```python
from build123d import *

# Parameters (mm, degrees)
SKETCH_1_W          = 80
SKETCH_1_H          = 36
EXTRUDE_1_DEPTH     = 2
CUT_EXTRUDE_1_DEPTH = 2
FILLET_2_R          = 2
SKETCH_3_R          = 1.5
CUT_EXTRUDE_2_DEPTH = 44.9089968


with BuildPart() as part:
    # 草图1 → 凸台-拉伸1 (new body)
    with BuildSketch(Plane.XY):
        Rectangle(SKETCH_1_W, SKETCH_1_H)
    extrude(amount=EXTRUDE_1_DEPTH)

    # 草图2 → 切除-拉伸1 (cut)
    with BuildSketch(Plane.XY.offset(2)):
        Polygon((-30, -8), (-30, -13), (30, -13), (30, -8), (30, 8), (30, 13), (-30, 13), (-30, 8), align=None)
    extrude(amount=-CUT_EXTRUDE_1_DEPTH, mode=Mode.SUBTRACT)

    # 圆角2
    fillet_2_edges = [part.edges().sort_by_distance(p)[0] for p in [
        (30, -13, 1),
        (-30, -13, 1),
        (-30, 13, 1),
        (30, 13, 1),
    ]]
    fillet(fillet_2_edges, radius=FILLET_2_R)

    # 草图3 → 切除-拉伸2 (cut, through all)
    with BuildSketch(Plane.XY.offset(2)):
        with Locations((23, -15)):
            Circle(SKETCH_3_R)
        with Locations((13, -15)):
            Circle(SKETCH_3_R)
        with Locations((-13, -15)):
            Circle(SKETCH_3_R)
        with Locations((-23, -15)):
            Circle(SKETCH_3_R)
        with Locations((23, 15)):
            Circle(SKETCH_3_R)
        with Locations((13, 15)):
            Circle(SKETCH_3_R)
        with Locations((-13, 15)):
            Circle(SKETCH_3_R)
        with Locations((-23, 15)):
            Circle(SKETCH_3_R)
    extrude(amount=-CUT_EXTRUDE_2_DEPTH, mode=Mode.SUBTRACT)


solid = part.part
```
Design review of the part built by this model. Coordinates are the model's own, in mm. A direction names the side the tool comes from. Coordinates: 2 decimals unless noted, no trailing zeros. Loops run counter-clockwise (first coordinate to the right, second up) from the corner with the lowest first, then second, coordinate; pieces in that order, holes last.
Q1. Tool access review of faces 4 (the face through (-29.4, -12.43, 0.99)), 5 (the face through (-1, -16, 0)): name each direction out of +Z, -Z, +X, -X, +Y, -Y from which nothing blocks a thin tool from reaching the whole face with its end or side.
Reported:
face 4: +Z, -Z
face 5: -Z, +X, -X, +Y, -Y
Q2. To check wall thickness, follow line 1 (Y direction, x = 13, z = 0.55); line 2 (Y direction, x = 27, z = 1.35); line 3 (X direction, y = -7, z = 1.3). State the ranges of each line that lie inside material, in increasing order.
Reported:
line 1: y = -18 to -16.5, -13.5 to -13, 13 to 13.5, 16.5 to 18
line 2: y = -18 to -13, 13 to 18
line 3: x = -40 to -30, 30 to 40
Q3. We need section D-D on y = -15. State the section outline as (x, z) points.
Reported:
outline: (-40, 0) - (-24.5, 0) - (-24.5, 2) - (-40, 2) - close; (-21.5, 0) - (-14.5, 0) - (-14.5, 2) - (-21.5, 2) - close; (-11.5, 0) - (11.5, 0) - (11.5, 2) - (-11.5, 2) - close; (14.5, 0) - (21.5, 0) - (21.5, 2) - (14.5, 2) - close; (24.5, 0) - (40, 0) - (40, 2) - (24.5, 2) - close
Q4. The part is to be moulded in two halves that separate along X. For faces 1 (the face through (-1, 18, 1)), 2 (the face through (40, 0, 1)), 3 (the face through (30, 0, 1)), say which applies: +X half, -X half, draft (parallel to the pull), parting line (faces both ways), or undercut.
Reported:
face 1: draft
face 2: +X half
face 3: undercut
Q5. We need section A-A on x = -23. State the section outline as (y, z) points.
Reported:
outline: (-18, 0) - (-16.5, 0) - (-16.5, 2) - (-18, 2) - close; (-13.5, 0) - (-13, 0) - (-13, 2) - (-13.5, 2) - close; (13, 0) - (13.5, 0) - (13.5, 2) - (13, 2) - close; (16.5, 0) - (18, 0) - (18, 2) - (16.5, 2) - close
Q6. We need section B-B on y = -9. State the section outline as (x, z) points.
Reported:
outline: (-40, 0) - (-30, 0) - (-30, 2) - (-40, 2) - close; (30, 0) - (40, 0) - (40, 2) - (30, 2) - close
Q7. We need section C-C on z = 0.85. State how many separate pieces and enclosed holes the cut face has, and give its area (3 significant figures).
Reported:
separate pieces: 1
enclosed holes: 9
area: 1,270 mm2
